```python
from build123d import *

# Parameters (mm, degrees)
F0_R     = 12
F1_DEPTH = 1
F2_R     = 2.5
F3_DEPTH = 1
F4_R     = 2
F5_DEPTH = 8
F6_R     = 2


with BuildPart() as f1:
    # F0 (on Top) → F1 (new body)
    with BuildSketch(Plane.XY):
        Circle(F0_R)
    extrude(amount=F1_DEPTH)

    # F2 (on Top) → F3 (join)
    with BuildSketch(Plane.XY):
        with Locations((-7.014924, 2.653458)):
            Circle(F2_R)
        with Locations((3.080317, -6.838249)):
            Circle(F2_R)
        with Locations((-3.085257, 6.836022)):
            Circle(F2_R)
        with Locations((-6.837136, -3.082787)):
            Circle(F2_R)
        Circle(F2_R)
        with Locations((6.839361, 3.077847)):
            Circle(F2_R)
        with Locations((7.013005, -2.658525)):
            Circle(F2_R)
        with Locations((-2.655992, -7.013965)):
            Circle(F2_R)
        with Locations((2.650924, 7.015882)):
            Circle(F2_R)
    extrude(amount=-F3_DEPTH)

    # F4 (on face) → F5 (join)
    with BuildSketch(Plane(origin=(0, 0, -1), x_dir=(1, 0, 0), z_dir=(0, 0, -1))):
        with Locations((-3.079479, -6.841555)):
            Circle(F4_R)
        with Locations((6.842186, -3.085332)):
            Circle(F4_R)
        Circle(F4_R)
        with Locations((2.650924, -7.015882)):
            Circle(F4_R)
        with Locations((-2.651925, 7.020854)):
            Circle(F4_R)
        with Locations((-7.02228, -2.650314)):
            Circle(F4_R)
        with Locations((3.08727, 6.842206)):
            Circle(F4_R)
        with Locations((7.019602, 2.663052)):
            Circle(F4_R)
        with Locations((-6.842561, 3.076908)):
            Circle(F4_R)
    extrude(amount=F5_DEPTH)

    # F6
    f6_edges = [f1.edges().sort_by_distance(p)[0] for p in [
        (-2, 0, -9),
        (-4.651925, -7.020854, -9),
        (0.650924, 7.015882, -9),
        (5.019602, -2.663052, -9),
        (-5.079479, 6.841555, -9),
        (4.842186, 3.085332, -9),
        (-9.02228, 2.650314, -9),
        (1.08727, -6.842206, -9),
        (-8.842561, -3.076908, -9),
    ]]
    fillet(f6_edges, radius=F6_R)


solid = f1.part
```
Source: CAD feature listing. Evaluate the final solid. Frame: model axes, mm. Round coordinates to 2 decimals unless told otherwise and drop trailing zeros. Loops run counter-clockwise (first coordinate to the right, second up) from the corner with the lowest first, then second, coordinate; pieces in that order, holes last. Notation, with made-up numbers: M -12.5,5 L 19.5,5 A21 ccw 19.5,40 Z; hole C -38.5,77 d11. An arc over 180 degrees is marked long. Use a Markdown table: item, result. Add a question column.
1. Section query A-A on z = -5.25. Give the number of separate pieces and of enclosed holes in the cut face, then the cut area to 3 significant figures.
2. Section query C-C on y = -1.5. Return the cut outline in (x, z), then the cut area to 3 significant figures.
3. Contact query for flat-ended pins moving along their axis: P1, Ø1.5, axis at x = -1.5, z = -1, coming from the +Y side; P2, Ø5, axis at y = 9, z = -8, coming from the -X side; P3, Ø1.5, axis at x = -3.5, y = -7.5, coming from the -Z side. Output: stop coordinate, or through.
4. Line query: line 1 (Z direction, x = -2, y = -3.75); line 2 (X direction, y = -6.5, z = -2.25); line 3 (Z direction, x = -8.75, y = -2.25). Output: solid intervals per line, ascending.
5. Section query B-B on x = -1.5. Return the cut outline in (y, z).
Reported:
| question | item | result |
|---|---|---|
| 1 | separate pieces | 9 |
| 1 | enclosed holes | 0 |
| 1 | area | 113 mm² |
| 2 | outline | M -11.91,0 L -8.77,0 L -8.77,-1 L -8.07,-1 L -8.07,-7 A1.23 ccw -5.61,-7 L -5.61,-1 L -4.9,-1 L -4.9,0 L -2,0 L -2,-1 L -1.32,-1 L -1.32,-7 A1.32 ccw 1.32,-7 L 1.32,-1 L 2,-1 L 2,0 L 4.8,0 L 4.8,-1 L 5.39,-1 L 5.39,-7 A1.63 ccw 8.65,-7 L 8.65,-1 L 9.23,-1 L 9.23,0 L 11.91,0 L 11.91,1 L -11.91,1 Z |
| 2 | area | 95.6 mm² |
| 3 | P1 | stops at y = 9.19 |
| 3 | P2 | stops at x = -5.08 |
| 3 | P3 | stops at z = -8.99 |
| 4 | line 1 | z = 0 to 1 |
| 4 | line 2 | x = -4.58 to -0.72, 1.12 to 5.06 |
| 4 | line 3 | z = -1 to 1 |
| 5 | outline | M -11.91,0 L -9.23,0 L -9.23,-1 L -8.66,-1 L -8.66,-7 A1.63 ccw -5.39,-7 L -5.39,-1 L -4.8,-1 L -4.8,0 L -2,0 L -2,-1 L -1.32,-1 L -1.32,-7 A1.32 ccw 1.32,-7 L 1.32,-1 L 2,-1 L 2,0 L 4.9,0 L 4.9,-1 L 5.61,-1 L 5.61,-7 A1.23 ccw 8.07,-7 L 8.07,-1 L 8.77,-1 L 8.77,0 L 11.91,0 L 11.91,1 L -11.91,1 Z |
